from build123d import *

# Parameters (mm, degrees)
F0_W     = 63.5
F0_H     = 38.1
F1_DEPTH = 25.4
F2_W     = 6.35
F2_H     = 34.925
F4_DEPTH = 7.9375
F3_W     = 15.875
F3_H     = 6.35
F5_DEPTH = 6.35
F6_DEPTH = 4.7625


# Not quite as in the source:
# - a length typed as a fraction of an inch, garbled in the dataset ("3 / 203.2 mm" for 3/8 in), is restored


with BuildPart() as f1:
    # F0 (on Top) → F1 (new body)
    with BuildSketch(Plane.XY):
        Rectangle(F0_W, F0_H)
    extrude(amount=F1_DEPTH)

    # F2 (on face) → F4 (cut)
    with BuildSketch(Plane.XY.offset(25.4)):
        with Locations((0, -1.5875)):
            Rectangle(F2_W, F2_H)
    extrude(amount=-F4_DEPTH, mode=Mode.SUBTRACT)

    # F3 (on face) → F5 (cut)
    with BuildSketch(Plane.XY.offset(25.4)):
        with Locations((11.1125, 11.1125)):
            Rectangle(F3_W, F3_H)
        with Locations((-11.1125, 11.1125)):
            Rectangle(F3_W, F3_H)
        with Locations((11.1125, -12.7)):
            Rectangle(F3_W, F3_H)
        with Locations((-11.1125, -12.7)):
            Rectangle(F3_W, F3_H)
    extrude(amount=-F5_DEPTH, mode=Mode.SUBTRACT)

    # F3 (on face) → F6 (cut)
    with BuildSketch(Plane.XY.offset(25.4)):
        with Locations((11.1125, -3.175)):
            Rectangle(F3_W, F3_H)
        with Locations((-11.1125, -3.175)):
            Rectangle(F3_W, F3_H)
    extrude(amount=-F6_DEPTH, mode=Mode.SUBTRACT)


solid = f1.part
Here's how the part is built. I have some questions about the finished solid (model axes, mm). A direction names the side the tool comes from. Coordinates: 2 decimals unless noted, no trailing zeros.
Item 1: On a 3-axis mill with a long thin cutter (end or side, diameter ignored), from which of +Z, -Z, +X, -X, +Y, -Y can I reach the whole of each face in a straight line? I mean faces 5 (the flat face through (-31.75, 0, 13)), 6 (the flat face through (-3.175, -2, 20)), 7 (the flat face through (11, -6.35, 23)). Say none if no direction works.
Item 2: Will this pin go through, and if not, where does the flat tip stop? pin 1 (1.9 mm diameter, centred on x = 11, y = -13.5, fed in from +Z).
Item 3: If we mould it in two halves opening along Y, with no side actions, what happens to faces 1 (the flat face through (-7.5, 0.3, 25.4)), 2 (the flat face through (11, 7.938, 22)), 3 (the flat face through (0, 15.875, 21)), 4 (the flat face through (-11, -6.35, 23))? For each: +Y half, -Y half, draft (parallel to the pull), parting line (faces both ways), or undercut.
Item 4: If I drill on line 1 (X direction, y = -11, z = 19) (3 decimals); line 2 (X direction, y = -10, z = 21.25); line 3 (Z direction, x = 4, y = 8), over which ranges is the centre line in solid material (lowest first)?
Findings below:
1. face 5: +Z, -Z, -X, +Y, -Y
1. face 6: +Z, -Y
1. face 7: +Z
2. pin 1: stops at z = 19.05
3. face 1: draft
3. face 2: undercut
3. face 3: -Y half
3. face 4: undercut
4. line 1: x = -31.75 to -3.175, 3.175 to 31.75
4. line 2: x = -31.75 to -19.05, 19.05 to 31.75
4. line 3: z = 0 to 19.05
